Design review of the part built by this model. Coordinates are the model's own, in mm. A direction names the side the tool comes from. Give positions to 0.01 mm unless a question says otherwise; leave off trailing zeros. Write each loop counter-clockwise with the first axis right and the second up, starting at its lowest first coordinate (ties: lowest second). Pieces come first, ordered by that corner, then holes. Notation, with made-up numbers: (5, 6.5) -> (39, 6.5) arc R19 ccw to (39, 30.5) -> close; hole circle Ø10 at (61, -32). An arc over 180 degrees is marked (long way). Use CSV: the item, a comma, the result in double quotes.
```python
from build123d import *

# Parameters (mm, degrees)
SKETCH_1_R      = 6.25
EXTRUDE_1_DEPTH = 3


with BuildPart() as part:
    # Эскиз1 → Бобышка-Вытянуть1 (new body)
    with BuildSketch(Plane.XY):
        with BuildLine():
            Line((-5.157518783, -12.8), (-4.45, -12.8))
            Line((-4.45, -12.8), (-4, -23.6))
            Line((-4, -23.6), (-1.65, -23.6))
            Line((-1.65, -23.6), (-1.65, -19))
            Line((-1.65, -19), (1.65, -19))
            Line((1.65, -19), (1.65, -23.6))
            Line((1.65, -23.6), (4, -23.6))
            Line((4, -23.6), (4.45, -12.8))
            Line((4.45, -12.8), (5.157518783, -12.8))
            ThreePointArc((5.157518783, -12.8), (13.798660493, 0.192272192), (4.79887218, 12.938733547))
            ThreePointArc((4.79887218, 12.938733547), (4.33946199, 12.880387443), (4.125, 12.469938853))
            Line((4.125, 12.469938853), (4.125, 8.185219421))
            Line((4.125, 8.185219421), (-4.125, 8.05))
            Line((-4.125, 8.05), (-4.125, 12.469938853))
            ThreePointArc((-4.125, 12.469938853), (-4.33946199, 12.880387443), (-4.79887218, 12.938733547))
            ThreePointArc((-4.79887218, 12.938733547), (-13.798660493, 0.192272192), (-5.157518783, -12.8))
        make_face()
        Circle(SKETCH_1_R, mode=Mode.SUBTRACT)
    extrude(amount=EXTRUDE_1_DEPTH)


solid = part.part
```
(1) Clearance check with flat-ended pins moving along their axes: pin 1 (1.5 mm diameter, centred on y = -21.5, z = 2, fed in from +X); pin 2 (0.9 mm diameter, centred on y = 11, z = 2, fed in from -X). State where each tip first meets the part, or that it passes through.
Established:
pin 1,"stops at x = 4.12"
pin 2,"stops at x = -8.9"
(2) Take a section at A-A (y = 0). Write out the cut boundary in (x, z), then the cut area to 3 significant figures.
Established:
outline,"(-13.8, 0) -> (-6.25, 0) -> (-6.25, 3) -> (-13.8, 3) -> close; (6.25, 0) -> (13.8, 0) -> (13.8, 3) -> (6.25, 3) -> close"
area,"45.3 mm2"
(3) Take a section at B-B (z = 1.65). Write out the cut boundary in (x, y) (3 decimals), then the cut area to 3 significant figures.
Established:
outline,"(-5.158, -12.8) -> (-4.45, -12.8) -> (-4, -23.6) -> (-1.65, -23.6) -> (-1.65, -19) -> (1.65, -19) -> (1.65, -23.6) -> (4, -23.6) -> (4.45, -12.8) -> (5.158, -12.8) arc R13.8 ccw to (4.799, 12.939) arc R0.5 ccw to (4.125, 12.47) -> (4.125, 8.185) -> (-4.125, 8.05) -> (-4.125, 12.47) arc R0.5 ccw to (-4.799, 12.939) arc R13.8 ccw to start; hole circle Ø12.5 at (0, 0)"
area,"499 mm2"
(4) Mouldability with a two-part tool opening along Y and no side actions: class faces 1 (the face through (4.22, -18.28, 1.48)), 2 (the face through (5.96, 1.88, 1.48)), 3 (the face through (13.8, 0, 1.5)) as +Y half, -Y half, draft (parallel to the pull), parting line (faces both ways), or undercut.
Established:
face 1,"-Y half"
face 2,"undercut"
face 3,"parting line"
(5) Tool access review of faces 4 (the face through (0, -9, 0)), 5 (the face through (4.125, 10, 1)), 6 (the face through (0, -19, 1)): name each direction out of +Z, -Z, +X, -X, +Y, -Y from which nothing blocks a thin tool from reaching the whole face with its end or side.
Established:
face 4,"-Z, +X, -X, +Y, -Y"
face 5,"+Z, -Z, +Y"
face 6,"+Z, -Z, -Y"
(6) For line 1 along Y through (x, z) = (-2.25, 2.05); line 2 along Y through (x, z) = (-1, 1.05); line 3 along X through (y, z) = (5, 1.4), list the stretches that pass through material, from the lowest coordinate up. Write a range as [from, to].
Established:
line 1,"y = [-23.6, -5.83], [5.83, 8.08]"
line 2,"y = [-19, -6.17], [6.17, 8.1]"
line 3,"x = [-12.86, -3.75], [3.75, 12.86]"
(7) Take a section at C-C (x = 0). Write out the cut boundary in (y, z), then the cut area to 3 significant figures.
Established:
outline,"(-19, 0) -> (-6.25, 0) -> (-6.25, 3) -> (-19, 3) -> close; (6.25, 0) -> (8.12, 0) -> (8.12, 3) -> (6.25, 3) -> close"
area,"43.9 mm2"
(8) Take a section at D-D (y = -12). Write out the cut boundary in (x, z), then the cut area to 3 significant figures.
Established:
outline,"(-6.81, 0) -> (6.81, 0) -> (6.81, 3) -> (-6.81, 3) -> close"
area,"40.9 mm2"
